CAD build for the part. Positions are in the model's coordinates, mm. A direction names the side the tool comes from. Round coordinates to 2 decimals unless told otherwise and drop trailing zeros. Order: outer loops, then holes, each group sorted by start corner. A loop starts at its lowest first (then second) coordinate and runs counter-clockwise, first axis right, second up. Notation, with made-up numbers: M 82.25,-4.5 L 101.25,-4.5 A31 cw 101.25,33.5 Z; hole C -11.75,-9.5 d7. An arc over 180 degrees is marked long. Put each result on its own line as item: value.
```python
from build123d import *

# Parameters (mm, degrees)
F2_W      = 76.2
F2_H      = 749.3
F3_DEPTH  = 76.2
F5_W      = 25.4
F5_H      = 150.9289524655
F6_DEPTH  = 76.2
F7_W      = 88.9
F7_H      = 109.3234665417
F8_DEPTH  = 13.2329911382
F10_W     = 121.5671412647
F10_H     = 124.9910257757
F11_DEPTH = 25.4
F13_W     = 25.4
F13_H     = 183.5729926825
F14_DEPTH = 76.2


with BuildPart() as f3:
    # F2 (on face) → F3 (new body)
    with BuildSketch(Plane(origin=(0, -0.2741353876, 1.5546990396), x_dir=(1, 0, 0), z_dir=(0, -0.1736481777, 0.984807753))):
        with Locations((-23.2936060824, -27.5516035191)):
            Rectangle(F2_W, F2_H)
    extrude(amount=F3_DEPTH)

    # F5 (on face) → F6 (cut)
    with BuildSketch(Plane.XZ.offset(-328.3190653867)):
        with Locations((-48.6936060824, 61.4055776064)):
            Rectangle(F5_W, F5_H)
        with Locations((2.1063939176, 61.4055776064)):
            Rectangle(F5_W, F5_H)
    extrude(amount=F6_DEPTH, mode=Mode.SUBTRACT)

    # F7 (on face) → F8 (cut, through all)
    with BuildSketch(Plane.XZ.offset(-328.3190653867)):
        with Locations((-16.9436060824, 94.7153790316)):
            Rectangle(F7_W, F7_H)
    extrude(amount=-F8_DEPTH, mode=Mode.SUBTRACT)

    # F10 (on face) → F11 (cut)
    with BuildSketch(Plane(origin=(0, -396.3653928071, 0), x_dir=(-1, 0, 0), z_dir=(0, 1, 0))):
        with Locations((6.2730181962, -37.5579986721)):
            Rectangle(F10_W, F10_H)
    extrude(amount=-F11_DEPTH, mode=Mode.SUBTRACT)

    # F13 (on face) → F14 (cut)
    with BuildSketch(Plane(origin=(0, -243.9653928071, 0), x_dir=(-1, 0, 0), z_dir=(0, 1, 0))):
        with Locations((23.2936060824, -0.4609301686)):
            Rectangle(F13_W, F13_H)
    extrude(amount=-F14_DEPTH, mode=Mode.SUBTRACT)


solid = f3.part
```
Item 1: Pin check, flat tips, straight feed: P1, Ø7.5, axis at x = -53, z = 103.5, coming from the +Y side; P2, Ø8, axis at x = -38.5, y = 246.5, coming from the +Z side; P3, Ø23, axis at y = 272.5, z = 87.5, coming from the -X side. Stop position of each tip, or through.
Answers below:
P1: y = 252.12
P2: z = 123.15
P3: x = -35.99
Item 2: Band-saw the part on C-C on z = 80.5. Give the cut face in (x, y).
Answers below:
outline: M -61.39,8.63 L 14.81,8.63 L 14.81,252.12 L -10.59,252.12 L -10.59,328.32 L -35.99,328.32 L -35.99,252.12 L -61.39,252.12 Z
Item 3: Band-saw the part on D-D on x = -54.5. Give the cut face in (y, z).
Answers below:
outline: M -396.37,-68.29 L 252.12,46.06 L 252.12,123.43 L -396.37,9.09 Z
Item 4: Mould opens along Y. For faces 6 (the flat face through (-23, 328.319, 99)), 7 (the flat face through (-23, -396.365, -29)), 8 (the flat face through (-10.594, -282, -10)) say: pulls with the +Y half, pulls with the -Y half, needs draft (parallel to the pull), parting line crosses it, or undercut.
Answers below:
face 6: pulls with the +Y half
face 7: pulls with the -Y half
face 8: undercut
Item 5: Probe line 1 along X through (y, z) = (-291, -39); line 2 along Z through (x, y) = (11, -170); line 3 along Z through (x, y) = (-2, 176). List the from-to ranges inside material, lowest first. Write a range as [from, to].
Answers below:
line 1: [-61.39, -35.99], [-10.59, 14.81]
line 2: [-28.37, 49]
line 3: [32.64, 110.01]
Item 6: Band-saw the part on A-A on x = -23. Give the cut face in (y, z), and give its area (3 significant figures).
Answers below:
outline: M -396.37,-68.29 L -320.17,-54.85 L -320.17,22.52 L -396.37,9.09 Z; M -243.97,-41.41 L 328.32,59.49 L 328.32,136.87 L -243.97,35.96 Z
area: 50,200 mm²
Item 7: Tool access for faces 1 (the flat face through (-23.83, -28.95, -3.5)), 2 (the flat face through (2, 252.119, 85)), 3 (the flat face through (-49, 252.119, 85)), 4 (the flat face through (14.806, -77, 26)), 5 (the flat face through (-35.994, -282, -10)): list every direction of +Z, -Z, +X, -X, +Y, -Y with a clear straight run to the whole face (end or side of a thin tool).
Answers below:
face 1: -Z, +X, -X, +Y
face 2: +Z, -Z, +X, +Y
face 3: +Z, -Z, -X, +Y
face 4: +Z, -Z, +X, +Y, -Y
face 5: +Z, -Z
Item 8: Band-saw the part on B-B on y = -292. Give the cut face in (x, z), and give its area (3 significant figures).
Answers below:
outline: M -61.39,-49.88 L -35.99,-49.88 L -35.99,27.49 L -61.39,27.49 Z; M -10.59,-49.88 L 14.81,-49.88 L 14.81,27.49 L -10.59,27.49 Z
area: 3,930 mm²
